Geometry: final body of the model. Coordinates: model frame, mm. A direction names the side the tool comes from. Coordinates: 2 decimals unless noted, no trailing zeros. Loops run counter-clockwise (first coordinate to the right, second up) from the corner with the lowest first, then second, coordinate; pieces in that order, holes last. Notation, with made-up numbers: (-32.75, 86) -> (-16.75, 86) arc R13 ccw to (-16.75, 96) -> close; hole circle Ø1 at (44, 45.25). An arc over 180 degrees is marked (long way). One line per item, written item: value. Start each with the question number.
Item 1: Section query C-C on x = 10. Return loops of the section in (y, z).
Item 2: Ray query, probe 1 along X at (y, z) = (1.8, 0); probe 2 along Z at (x, y) = (2.35, 35); probe 3 along Z at (x, y) = (11.5, 25). Return the intervals inside material, ascending. Write a range as from..to.
Item 3: Set-up query: faces 4 (the flat face through (3, 24, 0)), 5 (the flat face through (13, 13, -9)). Return all of +Z, -Z, +X, -X, +Y, -Y with unobstructed straight access to the full face (end or side cutting, diameter ignored); none if empty.
Item 4: Section query D-D on y = 28.5. Return loops of the section in (x, z).
Item 5: Section query A-A on x = 20. Return loops of the section in (y, z), then the cut area to 3 significant figures.
Item 6: Mould query, pull axis X, two halves, no side actions, for faces 1 (the cylindrical face through (38.47, 1.52, -0.46)), 2 (the flat face through (0, 22, 4)), 3 (the flat face through (13, 13, 9)). Classes: +X half, -X half, draft (parallel to the pull), parting line (faces both ways), or undercut.
Item 7: Contact query for flat-ended pins moving along their axis: pin 1 Ø4 at (x, z) = (20, 0) entering from -Y; pin 2 Ø1.5 at (y, z) = (14, -3) entering from +X; pin 3 Ø10 at (x, z) = (17.5, 0.5) entering from +Y; pin 4 Ø9 at (x, z) = (17.5, 2.5) entering from +Y. Output: stop coordinate, or through.
Item 8: Section query B-B on z = 7. Return loops of the section in (x, y), then the cut area to 3 significant figures.
from build123d import *

# Parameters (mm, degrees)
EXTRUDE_1_DEPTH     = 9
SHELL_START         = 3
SHELL_1_OUTLINE_W   = 37
SHELL_1_OUTLINE_H   = 12
SHELL_1_DEPTH       = 35
SKETCH_5_R          = 3.5
CUT_EXTRUDE_1_DEPTH = 63.20932406
SKETCH_6_R          = 3.5
CUT_EXTRUDE_2_DEPTH = 63.20932406
HOLE_WIZARD_M4_1_D  = 3.3


# Read off the part's stored shape, not the designer's step: 抽壳1
with BuildPart() as part:
    # 草图1 → 凸台-拉伸1 (new, symmetric)
    with BuildSketch(Plane.XY):
        Polygon((0, 0), (0, 45), (3, 45), (3, 38), (38, 3), (45, 3), (45, 0), align=None)
    extrude(amount=EXTRUDE_1_DEPTH, both=True)

    # 抽壳1 outline → 抽壳1 (cut)
    with BuildSketch(Plane(origin=(0, 0, 0), x_dir=(1, 0, 0), z_dir=(0, 1, 0)).offset(SHELL_START)):
        with Locations((21.5, 0)):
            Rectangle(SHELL_1_OUTLINE_W, SHELL_1_OUTLINE_H)
    extrude(amount=SHELL_1_DEPTH, mode=Mode.SUBTRACT)

    # 草图5 → 切除-拉伸1 (cut, through all)
    with BuildSketch(Plane(origin=(0, 3, 0), x_dir=(1, 0, 0), z_dir=(0, 1, 0))):
        with Locations(Location((20, 0, 0), (0, 0, 270))):
            Circle(SKETCH_5_R)
        with Locations(Location((35, 0, 0), (0, 0, 270))):
            Circle(SKETCH_5_R)
    extrude(amount=-CUT_EXTRUDE_1_DEPTH, mode=Mode.SUBTRACT)

    # 草图6 → 切除-拉伸2 (cut, through all)
    with BuildSketch(Plane(origin=(3, 0, 0), x_dir=(0, 0, -1), z_dir=(1, 0, 0))):
        with Locations(Location((0, 20, 0), (0, 0, 90))):
            Circle(SKETCH_6_R)
        with Locations(Location((0, 35, 0), (0, 0, 90))):
            Circle(SKETCH_6_R)
    extrude(amount=-CUT_EXTRUDE_2_DEPTH, mode=Mode.SUBTRACT)

    # M4 螺纹孔1 (through all)
    with Locations(Plane(origin=(0, 0, -9), x_dir=(-1, 0, 0), z_dir=(0, 0, -1))):
        with Locations((-10, 10)):
            Hole(HOLE_WIZARD_M4_1_D / 2)


solid = part.part
Reply:
1. outline: (0, -9) -> (8.35, -9) -> (8.35, -6) -> (3, -6) -> (3, 6) -> (8.35, 6) -> (8.35, 9) -> (0, 9) -> close; (11.65, -9) -> (31, -9) -> (31, -6) -> (11.65, -6) -> close; (11.65, 6) -> (31, 6) -> (31, 9) -> (11.65, 9) -> close
2. probe 1: x = 0..16.5, 23.5..31.5, 38.5..45
2. probe 2: z = -9..-3.5, 3.5..9
2. probe 3: z = -9..-6, 6..9
3. face 4: +X, +Y
3. face 5: -Z, +X, -X, +Y, -Y
4. outline: (0, -9) -> (12.5, -9) -> (12.5, -6) -> (3, -6) -> (3, 6) -> (12.5, 6) -> (12.5, 9) -> (0, 9) -> close
5. outline: (0, -9) -> (21, -9) -> (21, -6) -> (3, -6) -> (3, -3.5) -> (0, -3.5) -> close; (0, 3.5) -> (3, 3.5) -> (3, 6) -> (21, 6) -> (21, 9) -> (0, 9) -> close
5. area: 141 mm²
6. face 1: undercut
6. face 2: -X half
6. face 3: draft
7. pin 1: passes through
7. pin 2: stops at x = 3
7. pin 3: stops at y = 3
7. pin 4: stops at y = 26.33
8. outline: (0, 0) -> (45, 0) -> (45, 3) -> (38, 3) -> (3, 38) -> (3, 45) -> (0, 45) -> close; hole circle Ø3.3 at (10, 10)
8. area: 865 mm²
